from build123d import *

# Parameters (mm, degrees)
SKETCH_1_W      = 8
SKETCH_1_H      = 50
EXTRUDE_1_DEPTH = 1237.5
EXTRUDE_2_DEPTH = 8


with BuildPart() as part:
    # Эскиз1 → Бобышка-Вытянуть1 (new, symmetric)
    with BuildSketch(Plane.XY):
        Rectangle(SKETCH_1_W, SKETCH_1_H)
    extrude(amount=EXTRUDE_1_DEPTH, both=True)

    # Эскиз2 → Бобышка-Вытянуть2 (add)
    with BuildSketch(Plane(origin=(4, 0, 0), x_dir=(0, 0, -1), z_dir=(1, 0, 0))):
        with BuildLine():
            Line((-1237.5, -2.500000274), (-1237.5, 25))
            Line((-1237.5, 25), (-1260, 25))
            Line((-1260, 25), (-1260, 20))
            ThreePointArc((-1260, 20), (-1244.090097326, 13.40990248), (-1237.5, -2.500000274))
        make_face()
        with BuildLine():
            Line((-1237.5, -25), (-1237.5, -2.500000274))
            ThreePointArc((-1237.5, -2.500000274), (-1244.09009752, -18.409902674), (-1260, -25))
            Line((-1260, -25), (-1237.5, -25))
        make_face()
    extrude_2 = extrude(amount=-EXTRUDE_2_DEPTH)

    # Зеркальное отражение1: Бобышка-Вытянуть2 across plane
    add(extrude_2.mirror(Plane.XY))


solid = part.part
Check sheet for the modelled part. Datum: model origin and axes. Units: mm. Round coordinates to 2 decimals unless told otherwise and drop trailing zeros. Order: outer loops, then holes, each group sorted by start corner. A loop starts at its lowest first (then second) coordinate and runs counter-clockwise, first axis right, second up.
(1) Cross-section at A-A, the plane y = -14.5. Enter the section's corners in (x, z), and give its area (3 significant figures).
(2) Go/stop test with a flat-tipped pin: P1, Ø1, axis at x = 1.5, y = 12.5, coming from the -Z side. Record where the tip stops, or that it passes through.
(3) Scan lines: probe 1 along Z at (x, y) = (-3.5, -7); probe 2 along Z at (x, y) = (-1.25, 0). Record each from-to range of solid material in increasing order.
Check sheet entries:
1. outline: (-4, -1240.97) - (4, -1240.97) - (4, 1240.97) - (-4, 1240.97) - close
1. area: 19,900 mm2
2. P1: stops at z = -1243.69
3. probe 1: z = -1237.95 to 1237.95
3. probe 2: z = -1237.64 to 1237.64
